Check sheet for the drawn part. Datum: minimum x, y, z corner. Units: mm. A direction names the side the tool comes from. Round coordinates to 2 decimals unless told otherwise and drop trailing zeros. Write each loop counter-clockwise with the first axis right and the second up, starting at its lowest first coordinate (ties: lowest second). Pieces come first, ordered by that corner, then holes. Notation, with made-up numbers: (-14, -9) -> (-4, -9) arc R31 ccw to (-4, 16) -> close; hole circle Ø11 at (15.25, 71.5). An arc over 180 degrees is marked (long way). One line per item, written item: value. Start each with the question number.
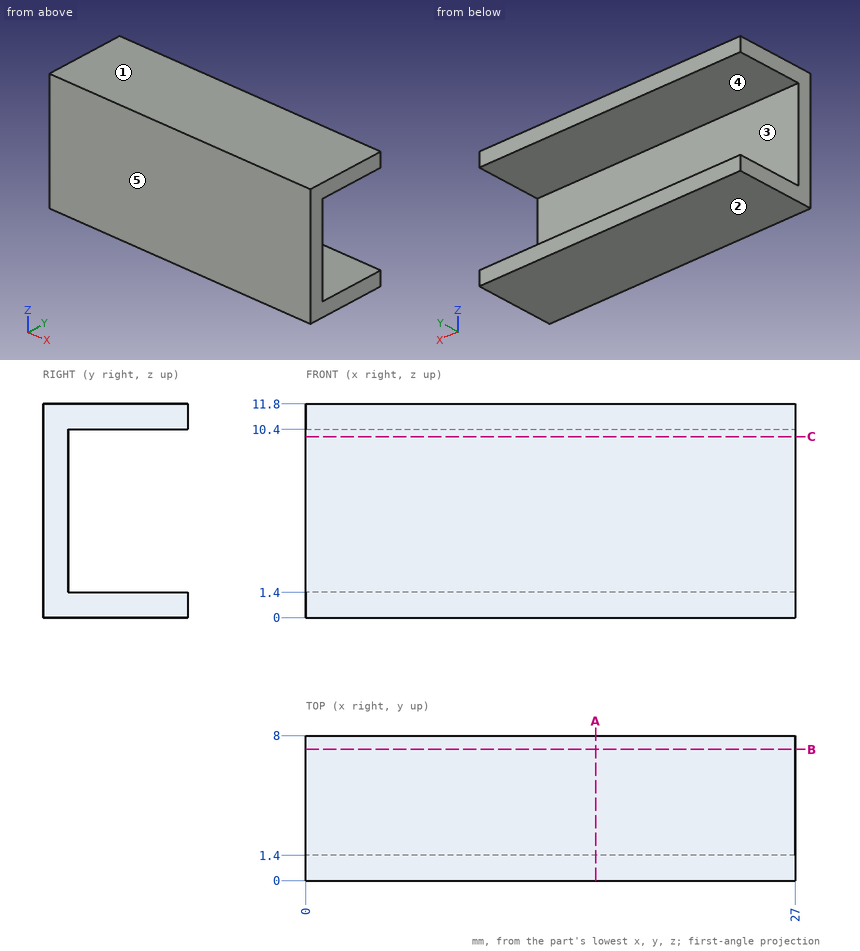
1. Cross-section at C-C (z = 10). Record the cut outline in (x, y).
2. Material ranges on probe 1 along Z at (x, y) = (21, 2.5); probe 2 along Y at (x, z) = (13.25, 8.75), recorded low to high.
3. Release check for a two-part mould opening along Z. For the marked faces 1, 2 and 3 record: +Z half, -Z half, draft (parallel to the pull), parting line (faces both ways), or undercut.
4. Cross-section at A-A (x = 16). Record the cut outline in (y, z).
5. Access from +Z, -Z, +X, -X, +Y, -Y to the whole of each face (thin tool, end or side, straight path). Record for the marked faces 4 and 5.
6. Depth check by flat-ended pin: pin 1 Ø3.5 at (x, y) = (16, 6) entering from -Z; pin 2 Ø2.5 at (x, z) = (19.5, 6) entering from +Y. Enter the tip coordinate at first touch or a pass-through.
7. Cross-section at B-B (y = 7.25). Record the cut outline in (x, z).
Working result:
1. outline: (0, 0) -> (27, 0) -> (27, 1.4) -> (0, 1.4) -> close
2. probe 1: z = 0 to 1.4, 10.4 to 11.8
2. probe 2: y = 0 to 1.4
3. face 1: +Z half
3. face 2: -Z half
3. face 3: undercut
4. outline: (0, 0) -> (8, 0) -> (8, 1.4) -> (1.4, 1.4) -> (1.4, 10.4) -> (8, 10.4) -> (8, 11.8) -> (0, 11.8) -> close
5. face 4: +X, -X, +Y
5. face 5: +Z, -Z, +X, -X, -Y
6. pin 1: stops at z = 0
6. pin 2: stops at y = 1.4
7. outline: (0, 0) -> (27, 0) -> (27, 1.4) -> (0, 1.4) -> close; (0, 10.4) -> (27, 10.4) -> (27, 11.8) -> (0, 11.8) -> close
